Design review of the part built by this model. Coordinates are the model's own, in mm. A direction names the side the tool comes from. Coordinates: 2 decimals unless noted, no trailing zeros. Order: outer loops, then holes, each group sorted by start corner. A loop starts at its lowest first (then second) coordinate and runs counter-clockwise, first axis right, second up. Notation, with made-up numbers: (-26.5, 43) - (-21.5, 43) arc R27 ccw to (-21.5, 79) - close; hole circle Ø4 at (-32.5, 42). An arc over 180 degrees is marked (long way). Write item = value, one per line. Start each with the question number.
```python
from build123d import *

# Parameters (mm, degrees)
F0_W     = 2.921
F0_H     = 25.4
F1_DEPTH = 2.54
F2_W     = 2.921
F2_H     = 25.4
F3_DEPTH = 10.16
F4_R     = 1.778
F5_DEPTH = 25.4


with BuildPart() as f1:
    # F0 (on Top) → F1 (new body)
    with BuildSketch(Plane.XY):
        Rectangle(F0_W, F0_H)
        with Locations((-2.921, 0)):
            Rectangle(F0_W, F0_H)
        with Locations((2.921, 0)):
            Rectangle(F0_W, F0_H)
    extrude(amount=F1_DEPTH)

    # F2 (on face) → F3 (join)
    with BuildSketch(Plane.XY.offset(2.54)):
        with Locations((-2.921, 0)):
            Rectangle(F2_W, F2_H)
        with Locations((2.921, 0)):
            Rectangle(F2_W, F2_H)
    extrude(amount=F3_DEPTH)

    # F4 (on face) → F5 (cut)
    with BuildSketch(Plane(origin=(-4.3815, 0, 0), x_dir=(0, -1, 0), z_dir=(-1, 0, 0))):
        with Locations((-6.35, 6.35)):
            Circle(F4_R)
        with Locations((6.35, 6.35)):
            Circle(F4_R)
    extrude(amount=-F5_DEPTH, mode=Mode.SUBTRACT)


solid = f1.part
```
Item 1: Mouldability with a two-part tool opening along X and no side actions: class faces 1 (the flat face through (0, 0, 2.54)), 2 (the cylindrical face through (2.9, 7.66, 7.55)), 3 (the flat face through (1.46, 0, 8)), 4 (the flat face through (-4.382, 0, 6)) as +X half, -X half, draft (parallel to the pull), parting line (faces both ways), or undercut.
Item 2: Add section B-B on y = -6.35. Give the boundary of the cut face in (x, z).
Item 3: For faces 5 (the flat face through (-1.46, 0, 8)), 6 (the cylindrical face through (-2.94, 7.66, 7.55)), list the 3-axis set-ups (+Z, -Z, +X, -X, +Y, -Y) from which the entire face can be reached by the end or side of a thin tool; tool diameter is ignored.
Item 4: Add section C-C on x = 3.5. Give the boundary of the cut face in (y, z), plus the area to 3 significant figures.
Item 5: For P1, Ø2, axis at y = -6.35, z = 6.35, coming from the +X side; P2, Ø1.5, axis at x = 0, y = -5, coming from the +Z side; P3, Ø2, axis at x = 2, y = -8.5, coming from the -Z side, all flat-tipped, find the tip position at first contact; note any pin that passes through.
Item 6: For line 1 (X direction, y = -0.5, z = 7.5); line 2 (Z direction, x = -2.45, y = -6.35); line 3 (Y direction, x = -3.25, z = 7.75), list the stretches that pass through material, from the lowest coordinate up.
Item 7: Add section D-D on z = 9.5. Give the boundary of the cut face in (x, y).
Item 8: Add section A-A on z = 6.35. Give the boundary of the cut face in (x, y), plus the area to 3 significant figures.
Worked out:
q1.face_1 = undercut
q1.face_2 = draft
q1.face_3 = undercut
q1.face_4 = -X half
q2.outline = (-4.38, 0) - (4.38, 0) - (4.38, 4.57) - (1.46, 4.57) - (1.46, 2.54) - (-1.46, 2.54) - (-1.46, 4.57) - (-4.38, 4.57) - close; (-4.38, 8.13) - (-1.46, 8.13) - (-1.46, 12.7) - (-4.38, 12.7) - close; (1.46, 8.13) - (4.38, 8.13) - (4.38, 12.7) - (1.46, 12.7) - close
q3.face_5 = +Z, +Y, -Y
q3.face_6 = +X, -X
q4.outline = (-12.7, 0) - (12.7, 0) - (12.7, 12.7) - (-12.7, 12.7) - close; hole circle Ø3.56 at (-6.35, 6.35); hole circle Ø3.56 at (6.35, 6.35)
q4.area = 303 mm2
q5.P1 = through
q5.P2 = 2.54
q5.P3 = 0
q6.line_1 = -4.38 to -1.46, 1.46 to 4.38
q6.line_2 = 0 to 4.57, 8.13 to 12.7
q6.line_3 = -12.7 to -7.45, -5.25 to 5.25, 7.45 to 12.7
q7.outline = (-4.38, -12.7) - (-1.46, -12.7) - (-1.46, 12.7) - (-4.38, 12.7) - close; (1.46, -12.7) - (4.38, -12.7) - (4.38, 12.7) - (1.46, 12.7) - close
q8.outline = (-4.38, -12.7) - (-1.46, -12.7) - (-1.46, -8.13) - (-4.38, -8.13) - close; (-4.38, -4.57) - (-1.46, -4.57) - (-1.46, 4.57) - (-4.38, 4.57) - close; (-4.38, 8.13) - (-1.46, 8.13) - (-1.46, 12.7) - (-4.38, 12.7) - close; (1.46, -12.7) - (4.38, -12.7) - (4.38, -8.13) - (1.46, -8.13) - close; (1.46, -4.57) - (4.38, -4.57) - (4.38, 4.57) - (1.46, 4.57) - close; (1.46, 8.13) - (4.38, 8.13) - (4.38, 12.7) - (1.46, 12.7) - close
q8.area = 107 mm2
